Here's how the part is built. I have some questions about the finished solid (model axes, mm). A direction names the side the tool comes from. Coordinates: 2 decimals unless noted, no trailing zeros. Write each loop counter-clockwise with the first axis right and the second up, starting at its lowest first coordinate (ties: lowest second). Pieces come first, ordered by that corner, then holes.
Item 1: I want a section at C-C (x = 5). Please give me the cut outline in (y, z).
Item 2: If we mould it in two halves opening along X, with no side actions, what happens to faces 5 (the face through (18, 4, 2)), 6 (the face through (0, 4, 2)), 7 (the face through (5.5, 6.4, 1.9)), 8 (the face through (5.5, -0.7, 1.8))? For each: pulls with the +X half, pulls with the -X half, needs draft (parallel to the pull), parting line crosses it, or undercut.
Item 3: I want a section at B-B (y = 2.5). Please give me the cut outline in (x, z).
Item 4: I want a section at A-A (y = 5.5). Please give me the cut outline in (x, z), and give its area (4 significant figures).
Item 5: I'm going to push flat-ended pins straight in: P1, Ø1, axis at y = -1, z = 1.5, coming from the -X side; P2, Ø1.5, axis at x = 11, y = 5.5, coming from the +Z side; P3, Ø0.7, axis at x = 17, z = 2, coming from the -Y side. Where does each tip first touch, or does it pass through?
Item 6: I want a section at D-D (y = 7.02). Please give me the cut outline in (x, z).
Item 7: Please list where these lines run through material, in increasing order: line 1 (X direction, y = -0.25, z = 1.35); line 2 (Y direction, x = 16.75, z = 2.2); line 3 (Z direction, x = 1.5, y = 7.02).
Item 8: For faces 1 (the face through (14.275, -2.507, 1.683)), 2 (the face through (1, 0, 2)), 3 (the face through (17, 0, 2)), 4 (the face through (8.951, 4.07, 2.975)), which set-ups out of +Z, -Z, +X, -X, +Y, -Y let a thin tool reach every point of the face, with its end or its side?
from build123d import *

# Parameters (mm, degrees)
BOSS_EXTRUDE2_DEPTH = 5
SKETCH8_R           = 50
CUT_EXTRUDE6_DEPTH  = 20
SKETCH9_OUTSIDE_W   = 10.609
SKETCH9_OUTSIDE_H   = 17.306
SKETCH9_OUTSIDE_R   = 50
CUT_EXTRUDE7_DEPTH  = 20
SKETCH11_W          = 2
SKETCH11_H          = 8
SKETCH11_W_2        = 7
BOSS_EXTRUDE4_DEPTH = 2
SKETCH12_OUTSIDE_W  = 9.573
SKETCH12_OUTSIDE_H  = 17.27
SKETCH12_OUTSIDE_R  = 50
CUT_EXTRUDE8_DEPTH  = 20
SKETCH13_R          = 0.3
CUT_EXTRUDE10_DEPTH = 20.924858845
SKETCH14_R          = 0.3
CUT_EXTRUDE11_DEPTH = 20
FILLET1_R           = 0.57


with BuildPart() as part:
    # Sketch1 → Boss-Extrude2 (new body)
    with BuildSketch(Plane.XY):
        Polygon((0, 0), (0, 8), (2, 8), (2, 5), (5.5, 6), (5.5, 8), (12.5, 8), (12.5, 6), (16, 5), (16, 8), (18, 8), (18, 0), (16, 0), (16, -3), (12.5, -2), (12.5, 0), (5.5, 0), (5.5, -2), (2, -3), (2, 0), align=None)
    extrude(amount=BOSS_EXTRUDE2_DEPTH)

    # Sketch8 → Cut-Extrude6 (cut)
    with BuildSketch(Plane(origin=(0, 0, 0), x_dir=(0, 0, -1), z_dir=(1, 0, 0))):
        with Locations((49, 2.5)):
            Circle(SKETCH8_R)
    extrude(amount=CUT_EXTRUDE6_DEPTH, mode=Mode.SUBTRACT)

    # Sketch9 outside → Cut-Extrude7 (cut)
    with BuildSketch(Plane(origin=(0, 0, 0), x_dir=(0, 0, -1), z_dir=(1, 0, 0))):
        with Locations((-2.8485, 2.5)):
            Rectangle(SKETCH9_OUTSIDE_W, SKETCH9_OUTSIDE_H)
        with Locations((47.1, 2.5)):
            Circle(SKETCH9_OUTSIDE_R, mode=Mode.SUBTRACT)
    extrude(amount=CUT_EXTRUDE7_DEPTH, mode=Mode.SUBTRACT)

    # Sketch11 → Boss-Extrude4 (add)
    with BuildSketch(Plane.XY.offset(4)):
        with Locations((1, 4)):
            Rectangle(SKETCH11_W, SKETCH11_H)
        with Locations((9, 4)):
            Rectangle(SKETCH11_W_2, SKETCH11_H)
        with Locations((17, 4)):
            Rectangle(SKETCH11_W, SKETCH11_H)
    extrude(amount=-BOSS_EXTRUDE4_DEPTH)

    # Sketch12 outside → Cut-Extrude8 (cut)
    with BuildSketch(Plane(origin=(0, 0, 0), x_dir=(0, 0, -1), z_dir=(1, 0, 0))):
        with Locations((-2.3485, 2.5)):
            Rectangle(SKETCH12_OUTSIDE_W, SKETCH12_OUTSIDE_H)
        with Locations((47, 2.5)):
            Circle(SKETCH12_OUTSIDE_R, mode=Mode.SUBTRACT)
    extrude(amount=CUT_EXTRUDE8_DEPTH, mode=Mode.SUBTRACT)

    # Sketch13 → Cut-Extrude10 (cut, through all)
    with BuildSketch(Plane(origin=(0, 0, 0), x_dir=(0, 0, -1), z_dir=(1, 0, 0))):
        with Locations(Location((-1.799307082, 7.02, 0), (0, 0, 270))):
            Circle(SKETCH13_R)
    extrude(amount=CUT_EXTRUDE10_DEPTH, mode=Mode.SUBTRACT)

    # Sketch14 → Cut-Extrude11 (cut)
    with BuildSketch(Plane(origin=(0, 0, 0), x_dir=(0, 0, -1), z_dir=(1, 0, 0))):
        with Locations(Location((-1.865607241, -1.2, 0), (0, 0, 270))):
            Circle(SKETCH14_R)
    extrude(amount=CUT_EXTRUDE11_DEPTH, mode=Mode.SUBTRACT)

    # Fillet1
    # the kernel refuses this fillet: 0.57 mm, written as the material it takes off along each edge
    with BuildSketch(Plane(origin=(19.370719987, 0, 2.937460889), x_dir=(0, 0, -1), z_dir=(-1, 0, 0))) as fillet1_piece_1:
        with BuildLine():
            CenterArc((0.545153795, -0.57), FILLET1_R, 90, 87.762310927)
            ThreePointArc((-0.024411551, -0.547744285), (-0.012956585, -0.273838681), (0, 0))
            Line((0, 0), (0.545153795, 0))
        make_face()
    extrude(amount=3.370719987, mode=Mode.SUBTRACT)
    with BuildSketch(Plane(origin=(19.28998783, 8, 2.696579359), x_dir=(0, 0, -1), z_dir=(-1, 0, 0)), Plane(origin=(3.28998783, 8, 2.696579359), x_dir=(0, 0, -1), z_dir=(-1, 0, 0))) as fillet1_piece_2:
        with BuildLine():
            CenterArc((0.513045529, 0.57), FILLET1_R, 185.724026079, 84.275973921)
            ThreePointArc((-0.054112356, 0.513149909), (-0.02771814, 0.25650515), (0, 0))
            Line((0, 0), (0.513045529, 0))
        make_face()
    extrude(amount=4.57997566, mode=Mode.SUBTRACT)
    with BuildSketch(Plane(origin=(12.5, 0, 2.937460889), x_dir=(0, 0, -1), z_dir=(-1, 0, 0))) as fillet1_piece_3:
        with BuildLine():
            CenterArc((0.545153795, -0.57), FILLET1_R, 90, 87.762310927)
            ThreePointArc((-0.024411551, -0.547744285), (-0.012956585, -0.273838681), (0, 0))
            Line((0, 0), (0.545153795, 0))
        make_face()
    extrude(amount=7, mode=Mode.SUBTRACT)
    with BuildSketch(Plane(origin=(13.78998783, 8, 2.696579359), x_dir=(0, 0, -1), z_dir=(-1, 0, 0))) as fillet1_piece_4:
        with BuildLine():
            CenterArc((0.513045529, 0.57), FILLET1_R, 185.724026079, 84.275973921)
            ThreePointArc((-0.054112356, 0.513149909), (-0.02771814, 0.25650515), (0, 0))
            Line((0, 0), (0.513045529, 0))
        make_face()
    extrude(amount=9.57997566, mode=Mode.SUBTRACT)
    with BuildSketch(Plane(origin=(2, 0, 2.937460889), x_dir=(0, 0.9990083494707687, 0.0445232263845563), z_dir=(-1, 0, 0))) as fillet1_piece_5:
        with BuildLine():
            CenterArc((0.545162753, 0.569991432), FILLET1_R, 182.551836528, 87.762310927)
            Line((-0.024272006, 0.544613193), (0, 0))
            ThreePointArc((0, 0), (0.274143997, -0.000751555), (0.548287995, 0))
        make_face()
    extrude(amount=3.370719987, mode=Mode.SUBTRACT)
    with BuildSketch(Plane(origin=(2, 0, 0.937460889), x_dir=(0, 0.9990278617443559, 0.04408323330360469), z_dir=(-1, 0, 0)), Plane(origin=(19.489241357, 0, 0.937460889), x_dir=(0, 0.9990278617443559, 0.04408323330360409), z_dir=(-1, 0, 0))) as fillet1_piece_6:
        with BuildLine():
            CenterArc((0.595706111, -0.569990001), FILLET1_R, 90.339381978, 92.187220026)
            Line((0.02626023, -0.595117444), (0, 0))
            ThreePointArc((0, 0), (0.296164915, -0.000877144), (0.592329831, 0))
        make_face()
    extrude(amount=3.489241357, mode=Mode.SUBTRACT)
    with BuildSketch(Plane(origin=(3.581343655, 8, 0.696579359), x_dir=(0, 0, 1), z_dir=(-1, 0, 0))) as fillet1_piece_7:
        with BuildLine():
            CenterArc((0.632537462, -0.57), FILLET1_R, 90, 95.594572842)
            ThreePointArc((0.065252578, -0.625568519), (0.033609947, -0.312681655), (0, 0))
            Line((0, 0), (0.632537462, 0))
        make_face()
    extrude(amount=5.16268731, mode=Mode.SUBTRACT)
    with BuildSketch(Plane(origin=(14.081343655, 8, 0.696579359), x_dir=(0, -0.9946037861150897, 0.1037463669027923), z_dir=(-1, 0, 0))) as fillet1_piece_8:
        with BuildLine():
            CenterArc((0.632547622, 0.569988725), FILLET1_R, 174.045055794, 95.594572842)
            Line((0.065623464, 0.629124155), (0, 0))
            ThreePointArc((0, 0), (0.314481268, 0.000988994), (0.628962535, 0))
        make_face()
    extrude(amount=10.16268731, mode=Mode.SUBTRACT)
    with BuildSketch(Plane(origin=(19.581343655, 8, 0.696579359), x_dir=(0, -0.9946037861150897, 0.1037463669027923), z_dir=(-1, 0, 0))) as fillet1_piece_9:
        with BuildLine():
            CenterArc((0.632547622, 0.569988725), FILLET1_R, 174.045055794, 95.594572842)
            Line((0.065623464, 0.629124155), (0, 0))
            ThreePointArc((0, 0), (0.314481268, 0.000988994), (0.628962535, 0))
        make_face()
    extrude(amount=5.16268731, mode=Mode.SUBTRACT)
    with BuildSketch(Plane(origin=(12.5, 0, 0.937460889), x_dir=(0, 0.9990278617443559, 0.04408323330360469), z_dir=(-1, 0, 0))) as fillet1_piece_10:
        with BuildLine():
            CenterArc((0.595706111, -0.569990001), FILLET1_R, 90.339381978, 92.187220026)
            Line((0.02626023, -0.595117444), (0, 0))
            ThreePointArc((0, 0), (0.296164915, -0.000877144), (0.592329831, 0))
        make_face()
    extrude(amount=7, mode=Mode.SUBTRACT)


solid = part.part
Answer:
1. outline: (-2.14, 0.78) arc R50 cw to (5.86, 0.89) - (5.86, 2.79) arc R50 ccw to (-2.14, 2.68) - close; hole circle Ø0.6 at (-1.2, 1.87)
2. face 5: pulls with the +X half
2. face 6: pulls with the -X half
2. face 7: undercut
2. face 8: undercut
3. outline: (0, 1) - (18, 1) - (18, 3) - (16, 3) - (16, 2.9) - (12.5, 2.9) - (12.5, 3) - (5.5, 3) - (5.5, 2.9) - (2, 2.9) - (2, 3) - (0, 3) - close
4. outline: (0, 0.91) - (2, 0.91) - (2, 2.91) - (0, 2.91) - close; (3.75, 0.91) - (14.25, 0.91) - (14.25, 2.81) - (12.5, 2.81) - (12.5, 2.91) - (5.5, 2.91) - (5.5, 2.81) - (3.75, 2.81) - close; (16, 0.91) - (18, 0.91) - (18, 2.91) - (16, 2.91) - close
4. area: 28.65 mm2
5. P1: stops at x = 2
5. P2: stops at z = 2.95
5. P3: stops at y = 0
6. outline: (0, 0.8) - (2, 0.8) - (2, 1.5) - (0, 1.5) - close; (0, 2.1) - (2, 2.1) - (2, 2.8) - (0, 2.8) - close; (5.5, 0.8) - (12.5, 0.8) - (12.5, 1.5) - (5.5, 1.5) - close; (5.5, 2.1) - (12.5, 2.1) - (12.5, 2.8) - (5.5, 2.8) - close; (16, 0.8) - (18, 0.8) - (18, 1.5) - (16, 1.5) - close; (16, 2.1) - (18, 2.1) - (18, 2.8) - (16, 2.8) - close
7. line 1: x = 2 to 5.5, 12.5 to 16
7. line 2: y = 0 to 8
7. line 3: z = 0.8 to 1.5, 2.1 to 2.8
8. face 1: +Z, -Z, -Y
8. face 2: +Z, -Z, -X, -Y
8. face 3: +Z, -Z, +X, -Y
8. face 4: +Z, +X, -X
